Geometry check sheet. Reference: the model listing, model coordinates, mm. Face numbers are marked on the shaded views. A direction names the side the tool comes from. Give positions to 0.01 mm unless a question says otherwise; leave off trailing zeros. Order: outer loops, then holes, each group sorted by start corner. A loop starts at its lowest first (then second) coordinate and runs counter-clockwise, first axis right, second up. Notation, with made-up numbers: M 2,68 L 27,68 A30 cw 27,93 Z; hole C -35,-38.75 d1. An arc over 180 degrees is marked long. Answer as CSV lines item,"result".
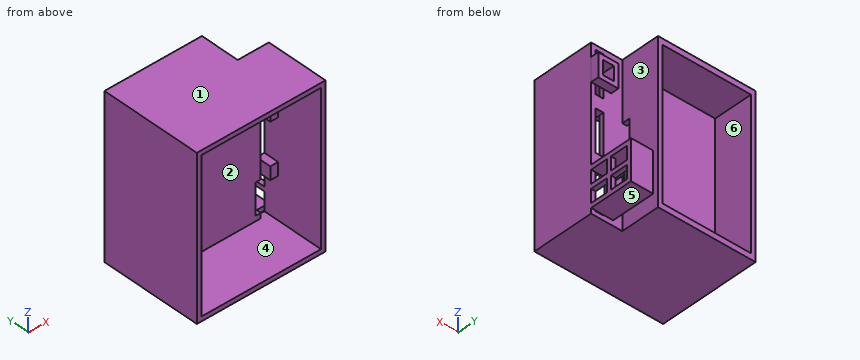
from build123d import *

# Parameters (mm, degrees)
SKETCH1_W               = 49.5
SKETCH1_H               = 61.5
BOSS_EXTRUDE1_DEPTH     = 23.75
SKETCH2_W               = 46
SKETCH2_H               = 58
CUT_EXTRUDE1_DEPTH      = 22
SKETCH3_W               = 3
SKETCH3_H               = 16
CUT_EXTRUDE2_DEPTH      = 1.75
SKETCH7_W               = 3
SKETCH7_H               = 5
BOSS_EXTRUDE2_DEPTH     = 4
SKETCH11_W              = 37.5
SKETCH11_H              = 61.5
BOSS_EXTRUDE3_DEPTH     = 15
SKETCH12_W              = 34
SKETCH12_H              = 57
CUT_EXTRUDE3_DEPTH      = 15
SKETCH14_W              = 7.75
SKETCH14_H              = 9
BOSS_EXTRUDE4_DEPTH     = 3
SKETCH15_W              = 4.25
SKETCH15_H              = 5.5
CUT_EXTRUDE4_DEPTH      = 4.75
SKETCH16_W              = 8.5
SKETCH16_H              = 15.5
BOSS_EXTRUDE5_DEPTH     = 16.75
SKETCH17_W              = 5.125
SKETCH17_H              = 6.625
CUT_EXTRUDE5_DEPTH      = 8.5
CUT_EXTRUDE6_DEPTH      = 15
CUT_EXTRUDE6_DEPTH_BACK = 1.75
SKETCH18_W              = 5
SKETCH18_H              = 12
SKETCH20_W              = 16
SKETCH20_H              = 3
CUT_EXTRUDE7_DEPTH      = 1.75


with BuildPart() as part:
    # Sketch1 → Boss-Extrude1 (new body)
    with BuildSketch(Plane(origin=(0, 0, 0), x_dir=(1, 0, 0), z_dir=(0, 1, 0))):
        with Locations((-113.412024913, -45.391200727)):
            Rectangle(SKETCH1_W, SKETCH1_H)
    extrude(amount=BOSS_EXTRUDE1_DEPTH)

    # Sketch2 → Cut-Extrude1 (cut)
    with BuildSketch(Plane(origin=(0, 0, 0), x_dir=(-1, 0, 0), z_dir=(0, -1, 0))):
        with Locations((113.412024913, -45.391200727)):
            Rectangle(SKETCH2_W, SKETCH2_H)
    extrude(amount=-CUT_EXTRUDE1_DEPTH, mode=Mode.SUBTRACT)

    # Sketch3 → Cut-Extrude2 (cut)
    with BuildSketch(Plane(origin=(0, 22, 0), x_dir=(-1, 0, 0), z_dir=(0, -1, 0))):
        with Locations((91.912024913, -66.391200727)):
            Rectangle(SKETCH3_W, SKETCH3_H)
        with Locations((91.912024913, -24.391200727)):
            Rectangle(SKETCH3_W, SKETCH3_H)
        with Locations((91.912024913, -45.391200727)):
            Rectangle(SKETCH3_W, SKETCH3_H)
    extrude(amount=-CUT_EXTRUDE2_DEPTH, mode=Mode.SUBTRACT)

    # Sketch7 → Boss-Extrude2 (add)
    with BuildSketch(Plane(origin=(0, 22, 0), x_dir=(-1, 0, 0), z_dir=(0, -1, 0))):
        with Locations((91.912024913, -55.891200727)):
            Rectangle(SKETCH7_W, SKETCH7_H)
        with Locations((91.912024913, -34.891200727)):
            Rectangle(SKETCH7_W, SKETCH7_H)
    extrude(amount=BOSS_EXTRUDE2_DEPTH)

    # Sketch11 → Boss-Extrude3 (add)
    with BuildSketch(Plane(origin=(0, 23.75, 0), x_dir=(1, 0, 0), z_dir=(0, 1, 0))):
        with Locations((-119.412024913, -45.391200727)):
            Rectangle(SKETCH11_W, SKETCH11_H)
    extrude(amount=BOSS_EXTRUDE3_DEPTH)

    # Sketch12 → Cut-Extrude3 (cut)
    with BuildSketch(Plane(origin=(0, 38.75, 0), x_dir=(1, 0, 0), z_dir=(0, 1, 0))):
        with Locations((-119.412024913, -45.391200727)):
            Rectangle(SKETCH12_W, SKETCH12_H)
    extrude(amount=-CUT_EXTRUDE3_DEPTH, mode=Mode.SUBTRACT)

    # Sketch14 → Boss-Extrude4 (add)
    with BuildSketch(Plane(origin=(0, 23.75, 0), x_dir=(1, 0, 0), z_dir=(0, 1, 0))):
        with Locations((-92.542024913, -66.391200727)):
            Rectangle(SKETCH14_W, SKETCH14_H)
    extrude(amount=BOSS_EXTRUDE4_DEPTH)

    # Sketch15 → Cut-Extrude4 (cut)
    with BuildSketch(Plane(origin=(0, 26.75, 0), x_dir=(1, 0, 0), z_dir=(0, 1, 0))):
        with Locations((-92.542024913, -66.391200727)):
            Rectangle(SKETCH15_W, SKETCH15_H)
    extrude(amount=-CUT_EXTRUDE4_DEPTH, mode=Mode.SUBTRACT)

    # Sketch16 → Boss-Extrude5 (add)
    with BuildSketch(Plane(origin=(0, 23.75, 0), x_dir=(1, 0, 0), z_dir=(0, 1, 0))):
        with Locations((-92.912024913, -24.391200727)):
            Rectangle(SKETCH16_W, SKETCH16_H)
    extrude(amount=BOSS_EXTRUDE5_DEPTH)

    # Sketch17 → Cut-Extrude5 (cut)
    with BuildSketch(Plane(origin=(-88.662024913, 0, 0), x_dir=(0, 0, -1), z_dir=(1, 0, 0))):
        with Locations((-27.828700727, 35.4375)):
            Rectangle(SKETCH17_W, SKETCH17_H)
        with Locations((-27.828700727, 27.0625)):
            Rectangle(SKETCH17_W, SKETCH17_H)
        with Locations((-20.953700727, 35.4375)):
            Rectangle(SKETCH17_W, SKETCH17_H)
        with Locations((-20.953700727, 27.0625)):
            Rectangle(SKETCH17_W, SKETCH17_H)
    extrude(amount=-CUT_EXTRUDE5_DEPTH, mode=Mode.SUBTRACT)

    # Sketch18 → Cut-Extrude6 (cut, two sides: drawn at the far end of the back side and taken through both)
    with BuildSketch(Plane(origin=(0, 23.75, 0), x_dir=(1, 0, 0), z_dir=(0, 1, 0)).offset(-CUT_EXTRUDE6_DEPTH_BACK)):
        with Locations((-92.912024913, -24.391200727)):
            Rectangle(SKETCH18_W, SKETCH18_H)
    extrude(amount=CUT_EXTRUDE6_DEPTH + CUT_EXTRUDE6_DEPTH_BACK, mode=Mode.SUBTRACT)

    # Sketch20 → Cut-Extrude7 (cut)
    with BuildSketch(Plane(origin=(-100.662024913, 0, 0), x_dir=(0, 0, -1), z_dir=(1, 0, 0))):
        with Locations((-45.391200727, 25.25)):
            Rectangle(SKETCH20_W, SKETCH20_H)
    extrude(amount=-CUT_EXTRUDE7_DEPTH, mode=Mode.SUBTRACT)


solid = part.part
(1) Tool access check on the marked faces 4, 5 and 6. Record the directions out of +Z, -Z, +X, -X, +Y, -Y that give a thin tool (end or side, any length) a straight path to the whole face; none if there is none.
The answers:
face 4,"-Y"
face 5,"-Z, +X, +Y"
face 6,"+Y"
(2) Material ranges on line 1 (X direction, y = 36.5, z = 22); line 2 (X direction, y = 11, z = 31); line 3 (X direction, y = 30.5, z = 22.5), recorded low to high.
The answers:
line 1,"x = -138.16 to -136.41, -102.41 to -100.66"
line 2,"x = -138.16 to -136.41, -90.41 to -88.66"
line 3,"x = -138.16 to -136.41, -102.41 to -100.66, -97.16 to -95.41, -90.41 to -88.66"
(3) Draft check along Z on the marked faces 1, 2 and 3. Enter one of: +Z half, -Z half, draft (parallel to the pull), parting line (faces both ways), or undercut.
The answers:
face 1,"+Z half"
face 2,"undercut"
face 3,"draft"
(4) Gauge pin test, flat ends, axial feed: P1, Ø1, axis at x = -127.5, z = 42, coming from the +Y side; P2, Ø1.9, axis at x = -96, y = 25.5, coming from the +Z side; P3, Ø1.4, axis at x = -96, y = 35.5, coming from the -Z side. Record the tip position at first contact, or that the pin passes through.
The answers:
P1,"stops at y = 23.75"
P2,"stops at z = 70.89"
P3,"stops at z = 16.64"
(5) Section check A-A on x = -91.5. State how many separate pieces and enclosed holes the cut face has, then the cut area to 3 significant figures.
The answers:
separate pieces,"7"
enclosed holes,"0"
area,"231 mm2"
(6) Section check B-B on z = 45. Enter the section's corners in (x, y), then the cut area to 3 significant figures.
The answers:
outline,"M -138.16,0 L -136.41,0 L -136.41,22 L -93.41,22 L -93.41,23.75 L -136.41,23.75 L -136.41,38.75 L -138.16,38.75 Z; M -102.41,26.75 L -100.66,26.75 L -100.66,38.75 L -102.41,38.75 Z; M -90.41,0 L -88.66,0 L -88.66,23.75 L -90.41,23.75 Z"
area,"206 mm2"
(7) Section check D-D on y = 3.5. Enter the section's corners in (x, z), then the cut area to 3 significant figures.
The answers:
outline,"M -138.16,14.64 L -88.66,14.64 L -88.66,76.14 L -138.16,76.14 Z; hole M -136.41,16.39 L -90.41,16.39 L -90.41,74.39 L -136.41,74.39 Z"
area,"376 mm2"
